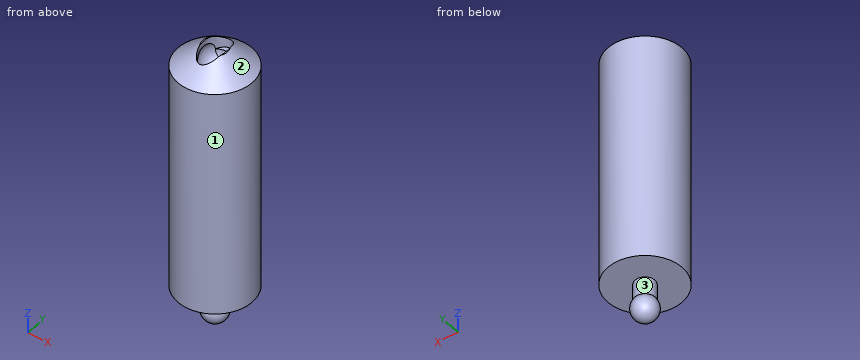
```python
from build123d import *

# Parameters (mm, degrees)
F0_R     = 7.5
F1_DEPTH = 50
F2_R     = 2
F3_DEPTH = 5
F7_DEPTH = 3


# Not quite as in the source:
# - a fillet or chamfer that OpenCascade refuses, or shapes differently, is made with other operations: its cross-section is extruded or revolved along the edge and cut away or added


with BuildPart() as f1:
    # F0 (on Top) → F1 (new body)
    with BuildSketch(Plane.XY):
        Circle(F0_R)
    extrude(amount=F1_DEPTH)

    # F2 (on face) → F3 (join)
    with BuildSketch(Plane(origin=(0, 0, 0), x_dir=(1, 0, 0), z_dir=(0, 0, -1))):
        Circle(F2_R)
    extrude(amount=F3_DEPTH)

    # F4 (on face) → F5 (revolve)
    with BuildSketch(Plane(origin=(0, 0, -5), x_dir=(1, 0, 0), z_dir=(0, 0, -1))):
        with BuildLine():
            Line((0, 2), (0, 2.5))
            ThreePointArc((0, 2.5), (-2.5, 0), (0, -2.5))
            Line((0, -2.5), (0, -2))
            ThreePointArc((0, -2), (-2, 0), (0, 2))
        make_face()
    revolve(axis=Axis((0, 0, -5), (0, 1, 0)))

    # F6 (on face) → F7 (cut)
    with BuildSketch(Plane.XY.offset(50)):
        with BuildLine():
            add(Edge.make_bspline(
                [(0, 4), (-3.897114317, 4), (-1.9485571585, -2), (0, -8), (1.9485571585, -2), (3.897114317, 4), (0, 4)],
                knots=[0, 0, 0, 2.0943951024, 2.0943951024, 4.1887902048, 4.1887902048, 6.2831853072, 6.2831853072, 6.2831853072], degree=2, weights=[1, 0.5, 1, 0.5, 1, 0.5, 1]))
        make_face()
    extrude(amount=-F7_DEPTH, mode=Mode.SUBTRACT)

    # F8 (on face) → F9 (revolve, cut)
    with BuildSketch(Plane.XY.offset(47)):
        with BuildLine():
            ThreePointArc((1.8, -2.4), (2.683281573, -1.3416407865), (3, 0))
            ThreePointArc((3, 0), (2.683281573, 1.3416407865), (1.8, 2.4))
            add(Edge.make_bspline(
                [(1.8, -2.4), (1.8810311774, -2.2079260981), (1.9485571585, -2), (2.6913429511, 0.2871870789), (1.8, 2.4)],
                knots=[4.0484923357, 4.0484923357, 4.0484923357, 4.1887902048, 4.1887902048, 5.3448576064, 5.3448576064, 5.3448576064], degree=2, weights=[0.9375, 0.9665063509, 1, 0.7240092377, 0.7527020789]))
        make_face()
        with BuildLine():
            Line((0, -3), (0, 3))
            ThreePointArc((0, 3), (-0.9486832981, 2.8460498942), (-1.8, 2.4))
            add(Edge.make_bspline(
                [(-1.8, 2.4), (-2.6913429511, 0.2871870789), (-1.9485571585, -2), (-1.8810311774, -2.2079260981), (-1.8, -2.4)],
                knots=[0.9383277008, 0.9383277008, 0.9383277008, 2.0943951024, 2.0943951024, 2.2346929715, 2.2346929715, 2.2346929715], degree=2, weights=[0.7527020789, 0.7240092377, 1, 0.9665063509, 0.9375]))
            ThreePointArc((-1.8, -2.4), (-0.9486832981, -2.8460498942), (0, -3))
        make_face()
    revolve(axis=Axis((0, 0, 47), (0, -1, 0)), mode=Mode.SUBTRACT)

    # F10: chamfer of 5 x 4 on 1 edges, made by hand

    # F10_s1 → F10_t2 (revolve, cut)
    with BuildSketch(Plane.XZ):
        Polygon((7.5, 46), (2.5, 50), (7.5, 50), align=None)
    revolve(axis=Axis((0, 0, 50), (0, 0, 1)), mode=Mode.SUBTRACT)


solid = f1.part
```
The listing builds one solid part. Answer for the finished solid, in the listing's coordinates (mm). Face numbers are marked on the shaded views. Give positions to 0.01 mm unless a question says otherwise; leave off trailing zeros. Write each loop counter-clockwise with the first axis right and the second up, starting at its lowest first coordinate (ties: lowest second). Pieces come first, ordered by that corner, then holes. Notation, with made-up numbers: M -5.5,-29.5 L 45.5,-29.5 A16 cw 45.5,-5.5 Z; hole C 47,0 d8. An arc over 180 degrees is marked long. Write each question's results on one line, items separated by ' | '.
Q1. For a pull along Z with two mould halves and no side action, classify the marked faces 1, 2 and 3 as released by +Z, released by -Z, zero draft, split by the parting line, or undercut.
Output values:
face 1: zero draft | face 2: released by +Z | face 3: undercut
Q2. Section A-A, the plane z = 40 is taken. Write down the section's boundary in (x, y), then the cut area to 3 significant figures.
Output values:
outline: C 0,0 d15 | area: 177 mm2
Q3. Consider L1, parallel to Y at x = 0.25, z = 17; L2, parallel to Y at x = 1.5, z = 45.5. Determine where each line is inside the solid, lowest interval first. Write a range as from..to.
Output values:
L1: -7.5..7.5 | L2: -7.35..-2.12, 2.12..7.35
Q4. Flat-ended cylindrical pins translate along their axes: P1, Ø2, axis at x = -0.5, y = 4, coming from the +Z side; P2, Ø1, axis at y = 4, z = 20.5, coming from the +X side; P3, Ø2, axis at x = -5.5, y = 0, coming from the +Z side. Find the tip coordinate at first contact, or state that the pin passes through.
Output values:
P1: z = 49.15 | P2: x = 6.63 | P3: z = 48.4
